```python
from build123d import *

# Parameters (mm, degrees)
BOSS_EXTRUDE1_DEPTH   = 7
BOSS_EXTRUDE1_2_DEPTH = 7
SKETCH2_R             = 4
SKETCH2_R_2           = 1.575
BOSS_EXTRUDE2_DEPTH   = 3
FILLET1_R             = 5
FILLET2_R             = 1
SKETCH3_R             = 6.014810067
SKETCH3_R_2           = 2.75
BOSS_EXTRUDE3_DEPTH   = 3
SKETCH4_R             = 2.5
CUT_EXTRUDE1_DEPTH    = 10


with BuildPart() as part:
    # Sketch1 → Boss-Extrude1 (new, symmetric)
    with BuildSketch(Plane.XY):
        with BuildLine():
            Line((-57.692807239, -27.704512139), (-71.0874428, -27.704512139))
            Line((-71.0874428, -27.704512139), (-54.981120944, -50))
            Line((-54.981120944, -50), (-39.949968711, -50))
            ThreePointArc((-39.949968711, -50), (-43.032344249, -47.373171188), (-45.942408988, -44.556649968))
            Line((-45.942408988, -44.556649968), (-48.76458719, -46.317700387))
            ThreePointArc((-48.76458719, -46.317700387), (-52.012858014, -46.915883336), (-54.794591341, -45.135140265))
            Line((-54.794591341, -45.135140265), (-60.064871871, -37.839652404))
            ThreePointArc((-60.064871871, -37.839652404), (-60.833011276, -34.338501535), (-58.79938816, -31.386811752))
            Line((-58.79938816, -31.386811752), (-56.544061175, -29.979478746))
            ThreePointArc((-56.544061175, -29.979478746), (-57.129759272, -28.847714043), (-57.692807239, -27.704512139))
        make_face()
    extrude(amount=BOSS_EXTRUDE1_DEPTH, both=True)



with BuildPart() as body_2:
    # Sketch1 → Boss-Extrude1 2 (new, symmetric)
    with BuildSketch(Plane.XY):
        with BuildLine():
            Line((39.949968711, -50), (54.981120944, -50))
            Line((54.981120944, -50), (71.0874428, -27.704512139))
            Line((71.0874428, -27.704512139), (57.692807239, -27.704512139))
            ThreePointArc((57.692807239, -27.704512139), (57.129759272, -28.847714043), (56.544061175, -29.979478746))
            Line((56.544061175, -29.979478746), (58.79938816, -31.386811752))
            ThreePointArc((58.79938816, -31.386811752), (60.833011276, -34.338501535), (60.064871871, -37.839652404))
            Line((60.064871871, -37.839652404), (54.794591341, -45.135140265))
            ThreePointArc((54.794591341, -45.135140265), (52.012858014, -46.915883336), (48.76458719, -46.317700387))
            Line((48.76458719, -46.317700387), (45.942408988, -44.556649968))
            ThreePointArc((45.942408988, -44.556649968), (43.032344249, -47.373171188), (39.949968711, -50))
        make_face()
    extrude(amount=BOSS_EXTRUDE1_2_DEPTH, both=True)


with BuildPart() as part_1:
    add(part.part)

    add(body_2.part)  # Boss-Extrude2 merges body 2
    # Sketch2 → Boss-Extrude2 (add)
    with BuildSketch(Plane.XY.offset(7)):
        Polygon((-54.981120944, -50), (54.981120944, -50), (71.0874428, -27.704512139), (-71.0874428, -27.704512139), align=None)
        with Locations((0, -41.25)):
            Circle(SKETCH2_R, mode=Mode.SUBTRACT)
        with Locations((-51.14684741, -42.5)):
            Circle(SKETCH2_R_2, mode=Mode.SUBTRACT)
        with Locations((-56.417127941, -35.204512139)):
            Circle(SKETCH2_R_2, mode=Mode.SUBTRACT)
        with Locations((56.417127941, -35.204512139)):
            Circle(SKETCH2_R_2, mode=Mode.SUBTRACT)
        with Locations((51.14684741, -42.5)):
            Circle(SKETCH2_R_2, mode=Mode.SUBTRACT)
    boss_extrude2 = extrude(amount=BOSS_EXTRUDE2_DEPTH)

    # Mirror2: Boss-Extrude2 across plane
    add(boss_extrude2.mirror(Plane.XY))

    # Fillet1
    fillet1_edges = [part_1.edges().sort_by_distance(p)[0] for p in [
        (-54.981120944, -50, 0),
        (-71.0874428, -27.704512139, 0),
        (54.981120944, -50, 0),
        (71.0874428, -27.704512139, 0),
    ]]
    fillet(fillet1_edges, radius=FILLET1_R)

    # Fillet2
    fillet2_edges = [part_1.edges().sort_by_distance(p)[0] for p in [
        (-39.949968711, -50, 0),
        (39.949968711, -50, 0),
    ]]
    fillet(fillet2_edges, radius=FILLET2_R)

    # Sketch3 → Boss-Extrude3 (add)
    with BuildSketch(Plane(origin=(0, 0, -10), x_dir=(-1, 0, 0), z_dir=(0, 0, -1))):
        with Locations((0, -41.25)):
            Circle(SKETCH3_R)
        with Locations((0, -41.25)):
            Circle(SKETCH3_R_2, mode=Mode.SUBTRACT)
    extrude(amount=-BOSS_EXTRUDE3_DEPTH)

    # Sketch4 → Cut-Extrude1 (cut)
    with BuildSketch(Plane.XY.offset(10)):
        with Locations((-25, -35.704512139)):
            Circle(SKETCH4_R)
        with Locations((25, -35.704512139)):
            Circle(SKETCH4_R)
    extrude(amount=-CUT_EXTRUDE1_DEPTH, mode=Mode.SUBTRACT)


solid = part_1.part
```
Can you work these out from the model? Positions are in its coordinate system, mm. A direction names the side the tool comes from. Give positions to 0.01 mm unless a question says otherwise; leave off trailing zeros. Loops run counter-clockwise (first coordinate to the right, second up) from the corner with the lowest first, then second, coordinate; pieces in that order, holes last. Notation, with made-up numbers: M 85,57 L 143,57 A7 ccw 143,62 Z; hole C 85,88 d2. An arc over 180 degrees is marked long. One line per item, written item: value.
(1) I need wall thicknesses on line 1 (Z direction, x = -18, y = -42.25); line 2 (Y direction, x = 0, z = -7.9); line 3 (X direction, y = -45, z = -1.5). Which ranges of each line are inside material? Lowest first, please.
Returned:
line 1: -10 to -7, 7 to 10
line 2: -50 to -44, -38.5 to -27.7
line 3: -58.59 to -54.89, -46.65 to -45.51, 45.51 to 46.65, 54.89 to 58.59
(2) Suppose I cut it at C-C on x = -6.5. List the corners of the cut face in (y, z) for me.
Returned:
outline: M -50,-10 L -27.7,-10 L -27.7,-7 L -50,-7 Z; M -50,7 L -27.7,7 L -27.7,10 L -50,10 Z
(3) Suppose I cut it at D-D on z = 8.75. List the corners of the cut face in (x, y) for me (3 decimals).
Returned:
outline: M -65.36,-35.632 L -56.478,-47.928 A5 ccw -52.425,-50 L 52.425,-50 A5 ccw 56.478,-47.928 L 65.36,-35.632 A5 ccw 61.307,-27.705 L -61.307,-27.705 A5 ccw Z; hole C -56.417,-35.205 d3.15; hole C -51.147,-42.5 d3.15; hole C -25,-35.705 d5; hole C 0,-41.25 d8; hole C 25,-35.705 d5; hole C 51.147,-42.5 d3.15; hole C 56.417,-35.205 d3.15
(4) We'd pull the mould along X, two halves only. Please class faces 4 (the face through (-1, -36, 10)), 5 (the face through (44.06, -46.42, 0.1)), 6 (the face through (54.671, -49.467, 0.14)): released by +X, released by -X, zero draft, split by the parting line, or undercut.
Returned:
face 4: zero draft
face 5: undercut
face 6: released by +X
(5) Suppose I cut it at A-A on x = -25. List the corners of the cut face in (y, z) for me, plus the area to 3 significant figures.
Returned:
outline: M -50,-10 L -27.7,-10 L -27.7,-7 L -50,-7 Z; M -50,7 L -38.2,7 L -38.2,10 L -50,10 Z; M -33.2,7 L -27.7,7 L -27.7,10 L -33.2,10 Z
area: 119 mm^2
(6) Suppose I cut it at B-B on y = -39.75. List the corners of the cut face in (x, z) for me, plus the area to 3 significant figures.
Returned:
outline: M -62.39,-10 L -2.3,-10 L -2.3,-7 L -58.68,-7 L -58.68,7 L -3.71,7 L -3.71,10 L -62.39,10 Z; M 2.3,-10 L 62.39,-10 L 62.39,10 L 3.71,10 L 3.71,7 L 58.68,7 L 58.68,-7 L 2.3,-7 Z
area: 816 mm^2
(7) Will these pins go through, and if not, where does the flat tip stop? pin 1 (10 mm diameter, centred on y = -38, z = 7.5, fed in from +X); pin 2 (10 mm diameter, centred on x = -39, z = 6.5, fed in from +Y); pin 3 (1.9 mm diameter, centred on x = -51.15, y = -42.5, fed in from -Z); pin 4 (4 mm diameter, centred on x = -25, y = -35.7, fed in from +Z).
Returned:
pin 1: x = 66.3
pin 2: y = -27.7
pin 3: through
pin 4: z = -7
(8) Which directions (+Z, -Z, +X, -X, +Y, -Y) give clear straight access to the entire face, cutting with the end or side of a thin tool? Please do faces 1 (the face through (-25.542, -38.145, 8.521)), 2 (the face through (-51.966, -46.925, 0.098)), 3 (the face through (-60.843, -34.389, 0.098)).
Returned:
face 1: +Z
face 2: +Y
face 3: none
